from build123d import *

# Parameters (mm, degrees)
SKETCH_1_W          = 18
SKETCH_1_H          = 18
EXTRUDE_1_DEPTH     = 1.5
CHAMFER_1_SIZE      = 1
SKETCH_2_W          = 18
SKETCH_2_H          = 12
EXTRUDE_2_DEPTH     = 1.5
CHAMFER_2_SIZE      = 1
CHAMFER_3_SIZE      = 1
CUT_EXTRUDE_2_DEPTH = 3
CHAMFER_5_SIZE      = 1
CUT_EXTRUDE_5_DEPTH = 3
EXTRUDE_12_DEPTH    = 2
EXTRUDE_13_DEPTH    = 2


with BuildPart() as part:
    # 草图1 → 凸台-拉伸1 (new body)
    with BuildSketch(Plane(origin=(0, 0, 0), x_dir=(1, 0, 0), z_dir=(0, 1, 0))):
        Rectangle(SKETCH_1_W, SKETCH_1_H)
    extrude(amount=EXTRUDE_1_DEPTH)

    # 倒角1
    chamfer_1_edges = [part.edges().sort_by_distance(p)[0] for p in [
        (0, 1.5, 9),
        (0, 1.5, -9),
    ]]
    chamfer(chamfer_1_edges, length=CHAMFER_1_SIZE)

    # 草图2 → 凸台-拉伸2 (add)
    with BuildSketch(Plane(origin=(0, 1.5, 0), x_dir=(1, 0, 0), z_dir=(0, 1, 0))):
        Rectangle(SKETCH_2_W, SKETCH_2_H)
    extrude(amount=EXTRUDE_2_DEPTH)

    # 倒角2
    chamfer_2_edges = [part.edges().sort_by_distance(p)[0] for p in [
        (0, 3, 6),
        (0, 3, -6),
    ]]
    chamfer(chamfer_2_edges, length=CHAMFER_2_SIZE)

    # 倒角3
    # the kernel refuses this chamfer: 1 mm, written as the material it takes off along each edge
    with BuildSketch(Plane(origin=(9, 1.5, 6), x_dir=(-0.9996219169112968, 0, 0.027495876610586487), z_dir=(0, 1, 0))) as chamfer_3_piece_1:
        Polygon((CHAMFER_3_SIZE * 0.999621916911, -CHAMFER_3_SIZE * 0.0274958766106), (-CHAMFER_3_SIZE * 0.0274958766106, -CHAMFER_3_SIZE * 0.999621916911), (0, 0), align=None)
    extrude(amount=3.071682988, mode=Mode.SUBTRACT)
    with BuildSketch(Plane(origin=(9, 1.5, 10.571682988), x_dir=(-0.9996219169112968, 0.02749587661058627, 0), z_dir=(0, 0, -1)), Plane(origin=(9, 1.5, -6), x_dir=(-0.9996219169112968, 0.02749587661058627, 0), z_dir=(0, 0, -1))) as chamfer_3_piece_2:
        Polygon((CHAMFER_3_SIZE * 0.999621916911, -CHAMFER_3_SIZE * 0.0274958766106), (-CHAMFER_3_SIZE * 0.0274958766106, -CHAMFER_3_SIZE * 0.999621916911), (0, 0), align=None)
    extrude(amount=4.571682988, mode=Mode.SUBTRACT)
    with BuildSketch(Plane(origin=(9, 1.5, -6), x_dir=(-0.9996219169112968, 0, -0.027495876610586535), z_dir=(0, 1, 0))) as chamfer_3_piece_3:
        Polygon((CHAMFER_3_SIZE * 0.999621916911, CHAMFER_3_SIZE * 0.0274958766106), (-CHAMFER_3_SIZE * 0.0274958766106, CHAMFER_3_SIZE * 0.999621916911), (0, 0), align=None)
    extrude(amount=3.071682988, mode=Mode.SUBTRACT)
    with BuildSketch(Plane(origin=(9, 3, -7.571682988), x_dir=(-0.9996219169112968, 0.027495876610586487, 0), z_dir=(0, 0, 1))) as chamfer_3_piece_4:
        Polygon((CHAMFER_3_SIZE * 0.999621916911, CHAMFER_3_SIZE * 0.0274958766106), (-CHAMFER_3_SIZE * 0.0274958766106, CHAMFER_3_SIZE * 0.999621916911), (0, 0), align=None)
    extrude(amount=15.143365976, mode=Mode.SUBTRACT)
    with BuildSketch(Plane(origin=(9, -1.071682988, 6), x_dir=(-0.9996219169112968, 0, 0.027495876610586487), z_dir=(0, 1, 0))) as chamfer_3_piece_5a_section:
        Polygon((CHAMFER_3_SIZE * 0.999621916911, -CHAMFER_3_SIZE * 0.0274958766106), (-CHAMFER_3_SIZE * 0.0274958766106, -CHAMFER_3_SIZE * 0.999621916911), (0, 0), align=None)
    chamfer_3_piece_5a = extrude(amount=5.643365976, mode=Mode.PRIVATE)
    chamfer_3_piece_5a = split(chamfer_3_piece_5a, bisect_by=Plane(origin=(8.670206373, 1.5, 5.670206373), z_dir=(0, -1, 0)), keep=Keep.TOP, mode=Mode.PRIVATE)
    with BuildSketch(Plane(origin=(9, 1.5, 10.571682988), x_dir=(-0.9996219169112968, 0.02749587661058627, 0), z_dir=(0, 0, -1))) as chamfer_3_piece_5b_section:
        Polygon((CHAMFER_3_SIZE * 0.999621916911, -CHAMFER_3_SIZE * 0.0274958766106), (-CHAMFER_3_SIZE * 0.0274958766106, -CHAMFER_3_SIZE * 0.999621916911), (0, 0), align=None)
    chamfer_3_piece_5b = extrude(amount=7.143365976, mode=Mode.PRIVATE)
    chamfer_3_piece_5b = split(chamfer_3_piece_5b, bisect_by=Plane(origin=(8.670206373, 1.170206373, 6), z_dir=(0, 0, -1)), keep=Keep.TOP, mode=Mode.PRIVATE)
    chamfer_3_piece_5 = chamfer_3_piece_5a & chamfer_3_piece_5b
    add(chamfer_3_piece_5, mode=Mode.SUBTRACT)
    with BuildSketch(Plane(origin=(9, -1.071682988, -6), x_dir=(-0.9996219169112968, 0, -0.027495876610586487), z_dir=(0, 1, 0))) as chamfer_3_piece_6a_section:
        Polygon((CHAMFER_3_SIZE * 0.999621916911, CHAMFER_3_SIZE * 0.0274958766106), (-CHAMFER_3_SIZE * 0.0274958766106, CHAMFER_3_SIZE * 0.999621916911), (0, 0), align=None)
    chamfer_3_piece_6a = extrude(amount=5.643365976, mode=Mode.PRIVATE)
    chamfer_3_piece_6a = split(chamfer_3_piece_6a, bisect_by=Plane(origin=(8.670206373, 1.5, -5.670206373), z_dir=(0, -1, 0)), keep=Keep.TOP, mode=Mode.PRIVATE)
    with BuildSketch(Plane(origin=(9, 1.5, -3.428317012), x_dir=(-0.9996219169112968, 0.02749587661058627, 0), z_dir=(0, 0, -1))) as chamfer_3_piece_6b_section:
        Polygon((CHAMFER_3_SIZE * 0.999621916911, -CHAMFER_3_SIZE * 0.0274958766106), (-CHAMFER_3_SIZE * 0.0274958766106, -CHAMFER_3_SIZE * 0.999621916911), (0, 0), align=None)
    chamfer_3_piece_6b = extrude(amount=7.143365976, mode=Mode.PRIVATE)
    chamfer_3_piece_6b = split(chamfer_3_piece_6b, bisect_by=Plane(origin=(8.670206373, 1.170206373, -6), z_dir=(0, 0, 1)), keep=Keep.TOP, mode=Mode.PRIVATE)
    chamfer_3_piece_6 = chamfer_3_piece_6a & chamfer_3_piece_6b
    add(chamfer_3_piece_6, mode=Mode.SUBTRACT)

    # 草图9 → 切除-拉伸2 (cut)
    with BuildSketch(Plane.ZY.offset(9)):
        Polygon((-6, 1.5), (-6, 2), (-5, 3), (5, 3), (6, 2), (6, 1.5), align=None)
    extrude(amount=-CUT_EXTRUDE_2_DEPTH, mode=Mode.SUBTRACT)

    # 倒角5
    chamfer_5_edges = [part.edges().sort_by_distance(p)[0] for p in [
        (-6, 3, 0),
    ]]
    chamfer(chamfer_5_edges, length=CHAMFER_5_SIZE)

    # 草图23 → 切除-拉伸5 (cut)
    with BuildSketch(Plane.ZY.offset(9)):
        Polygon((9, 0.5), (8, 1.5), (-8, 1.5), (-9, 0.5), (-9, 0), (9, 0), align=None)
    extrude(amount=-CUT_EXTRUDE_5_DEPTH, mode=Mode.SUBTRACT)

    # 草图24 → 凸台-拉伸12 (add)
    with BuildSketch(Plane(origin=(0, 0, -6), x_dir=(-1, 0, 0), z_dir=(0, 0, -1))):
        Polygon((6, 1.5), (4, 2), (-8, 2), (-8, 1.5), align=None)
    extrude(amount=EXTRUDE_12_DEPTH)

    # 草图25 → 凸台-拉伸13 (add)
    with BuildSketch(Plane.XY.offset(6)):
        Polygon((-6, 1.5), (-4, 2), (8, 2), (8, 1.5), align=None)
    extrude(amount=EXTRUDE_13_DEPTH)


solid = part.part
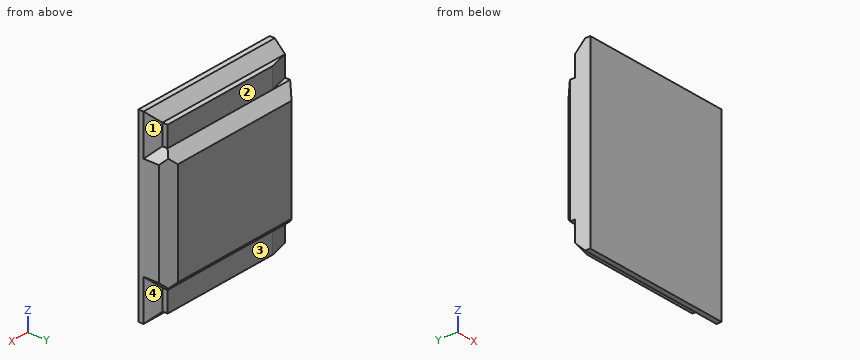
Design review of the part built by this model. Coordinates are the model's own, in mm. Face numbers are marked on the shaded views. A direction names the side the tool comes from. Coordinates: 2 decimals unless noted, no trailing zeros. Order: outer loops, then holes, each group sorted by start corner. A loop starts at its lowest first (then second) coordinate and runs counter-clockwise, first axis right, second up. Notation, with made-up numbers: (67.5, 64) - (92.5, 64) arc R30 cw to (92.5, 99) - close; hole circle Ø6 at (6.5, -33.75). An arc over 180 degrees is marked (long way). Put each result on its own line as item: value.
1) Take a section at A-A, the plane y = 0.7. Give the boundary of the cut face in (x, z), and give its area (3 significant figures).
Response values:
outline: (-6, -8.8) - (8.8, -8.8) - (8.8, -5.2) - (9, -5) - (9, 5) - (8.8, 5.2) - (8.8, 8.8) - (-6, 8.8) - close
area: 263 mm²
2) Wall thickness on L1, parallel to Z at x = 4.5, y = 1.95; L2, parallel to Z at x = -1, y = 0.9; L3, parallel to X at y = 2.8, z = 2.5: over which ranges is each line inside the solid? List them lowest first. Write a range as from..to.
Response values:
L1: z = -8..8
L2: z = -8.6..8.6
L3: x = -5.2..8.2
3) Take a section at D-D, the plane y = 2.25. Give the boundary of the cut face in (x, z).
Response values:
outline: (-5.75, -5.75) - (8.25, -5.75) - (8.75, -5.25) - (8.75, 5.25) - (8.25, 5.75) - (-5.75, 5.75) - close
4) Tool access review of the marked faces 1, 2, 3 and 4: name each direction out of +Z, -Z, +X, -X, +Y, -Y from which nothing blocks a thin tool from reaching the whole face with its end or side.
Response values:
face 1: +Z, +X, +Y
face 2: +Z, +X, -X, +Y
face 3: -Z, +X, -X, +Y
face 4: -Z, +X, +Y
5) Insertion check: P1, Ø2, axis at x = 2, z = 7.5, coming from the +Y side. The pin has a flat end and moves straight along its axis. Give the tip position at first contact, or say it passes through.
Response values:
P1: stops at y = 2
6) Take a section at B-B, the plane x = 7. Give the boundary of the cut face in (y, z).
Response values:
outline: (0, -9) - (0.5, -9) - (1.5, -8) - (2, -8) - (2, -6) - (3, -5) - (3, 5) - (2, 6) - (2, 8) - (1.5, 8) - (0.5, 9) - (0, 9) - close
7) Take a section at C-C, the plane z = 3.75. Give the boundary of the cut face in (x, y).
Response values:
outline: (-6, 0) - (9, 0) - (9, 2) - (8, 3) - (-5, 3) - (-6, 2) - close
